Here's the drawing with two shaded views (mm, measured from the low corner). I have some questions. A direction names the side the tool comes from. Give positions to 0.01 mm unless a question says otherwise; leave off trailing zeros. Order: outer loops, then holes, each group sorted by start corner. A loop starts at its lowest first (then second) coordinate and runs counter-clockwise, first axis right, second up. Notation, with made-up numbers: (25, 25) - (76, 25) arc R24 ccw to (76, 36) - close; hole circle Ø2 at (-24.75, 38). An arc over 180 degrees is marked (long way). Use one line per item in the form item = value. Start each with the question number.
1) Suppose I cut it at A-A, the plane y = 5.75. Write out the boundary of the cut face in (x, z), and give its area (3 significant figures).
2) Suppose I cut it at B-B, the plane x = 59. Write out the boundary of the cut face in (y, z) (1 decimal).
3) Please list where these lines run through material, in increasing order: probe 1 along Z at (x, y) = (69.85, 20.25); probe 2 along Z at (x, y) = (69.85, 2.75).
4) Which directions (+Z, -Z, +X, -X, +Y, -Y) give clear straight access to the entire face, cutting with the end or side of a thin tool? Please do the marked faces 4 and 5.
5) Suppose I cut it at D-D, the plane y = 20.5. Write out the boundary of the cut face in (x, z).
6) For pin 1 (2 mm diameter, centred on x = 50.5, z = 82, fed in from -Y) (3 decimals); pin 2 (10 mm diameter, centred on y = 23, z = 40.5, fed in from +X); pin 3 (1 mm diameter, centred on x = 68.5, y = 21, fed in from -Z); pin 4 (2 mm diameter, centred on x = 69.85, z = 69.85, fed in from -Y), each with a flat end and sliding along its axis, tell me the tip position at first contact or that it passes through.
7) Suppose I cut it at C-C, the plane z = 62.5. Write out the boundary of the cut face in (x, y) (1 decimal).
8) We'd pull the mould along X, two halves only. Please class the marked faces 1, 2 and 3: released by +X, released by -X, zero draft, split by the parting line, or undercut.
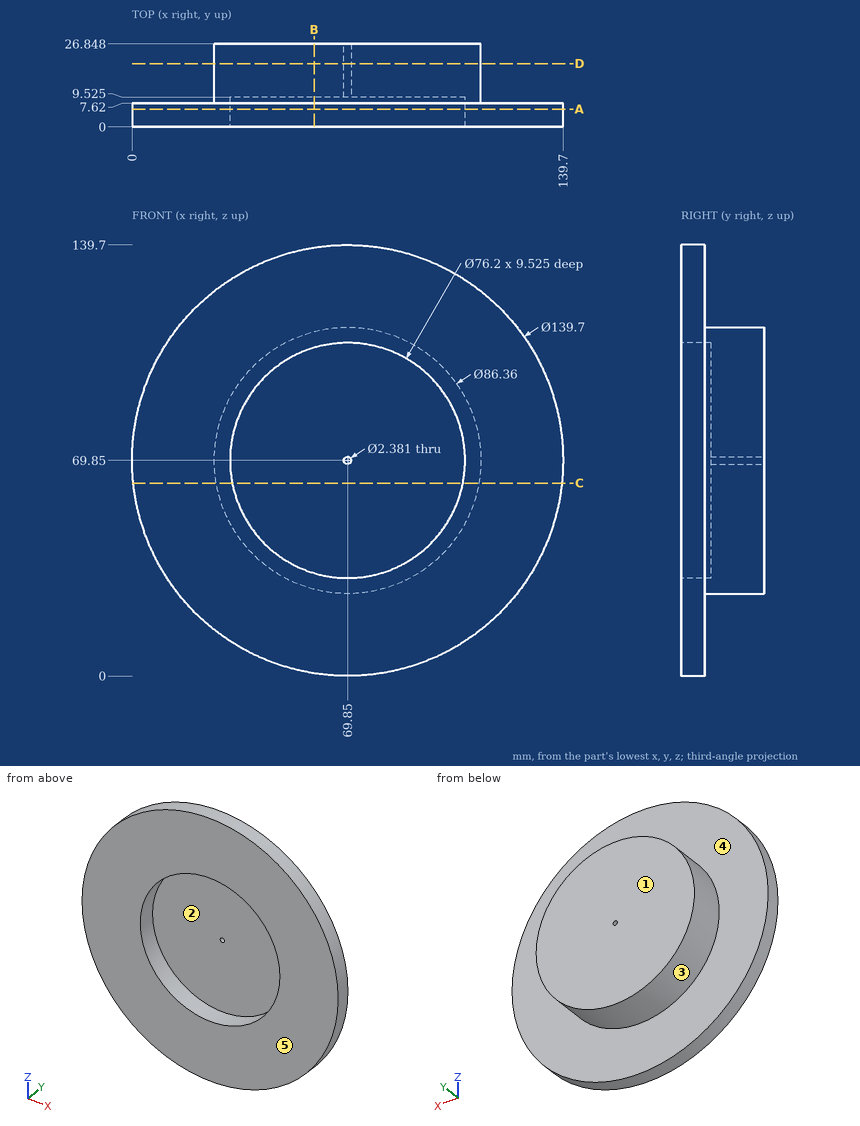
Result sheet:
q1.outline = circle Ø139.7 at (69.85, 69.85); hole circle Ø76.2 at (69.85, 69.85)
q1.area = 10,800 mm²
q2.outline = (0, 0.8) - (7.6, 0.8) - (7.6, 28.1) - (26.8, 28.1) - (26.8, 111.6) - (7.6, 111.6) - (7.6, 138.9) - (0, 138.9) - (0, 106.4) - (9.5, 106.4) - (9.5, 33.3) - (0, 33.3) - close
q3.probe_1 = 26.67 to 68.66, 71.04 to 113.03
q3.probe_2 = 0 to 31.75, 107.95 to 139.7
q4.face_4 = +Y
q4.face_5 = +Z, -Z, +X, -X, -Y
q5.outline = circle Ø86.36 at (69.85, 69.85); hole circle Ø2.38 at (69.85, 69.85)
q6.pin_1 = 9.525
q6.pin_2 = 105.51
q6.pin_3 = 26.68
q6.pin_4 = through
q7.outline = (0.4, 0) - (32.5, 0) - (32.5, 9.5) - (107.2, 9.5) - (107.2, 0) - (139.3, 0) - (139.3, 7.6) - (112.4, 7.6) - (112.4, 26.8) - (27.3, 26.8) - (27.3, 7.6) - (0.4, 7.6) - close
q8.face_1 = zero draft
q8.face_2 = undercut
q8.face_3 = split by the parting line
